Model file for the job. Use its own axes, mm. Give positions to 0.01 mm unless a question says otherwise; leave off trailing zeros. Order: outer loops, then holes, each group sorted by start corner. A loop starts at its lowest first (then second) coordinate and runs counter-clockwise, first axis right, second up. Notation, with made-up numbers: M 88,88 L 112,88 A25 ccw 112,111 Z; hole C -21.75,56.5 d1. An arc over 180 degrees is marked long. Return JSON: item names as keys, results as strings. Group by question number.
1. Slice it at B-B on z = 0. List the corners of the cut face in (x, y).
2. Slice it at D-D on z = -10. List the corners of the cut face in (x, y), then the cut area to 3 significant figures.
3. Pin check, flat tips, straight feed: pin 1 (2 mm diameter, centred on x = -8, y = -11.5, fed in from -Z); pin 2 (2.5 mm diameter, centred on x = -3.94, z = 6.82, fed in from +Y); pin 3 (4 mm diameter, centred on x = 4, y = -14.5, fed in from +Z); pin 4 (1 mm diameter, centred on y = -12, z = -9, fed in from -X). Stop position of each tip, or through.
4. Wall check: probe 1 along Z at (x, y) = (-3.25, -6.5); probe 2 along Z at (x, y) = (-2.75, -8.75); probe 3 along X at (y, z) = (-14.25, 5.75). Give the ranges that are in metal, low to high. Write a range as [from, to].
5. Slice it at C-C on x = 10.5. List the corners of the cut face in (y, z), then the cut area to 3 significant figures.
6. Two-plate mould, pull along X, no slides. Class faces 1 (the face through (-3.131, -10.14, 8.085)), 2 (the face through (-7.246, -9.86, 10.186)), 3 (the face through (6.377, -10.14, 0.066)), 4 (the face through (5.199, -9.86, 11.368)): released by +X, released by -X, zero draft, split by the parting line, or undercut.
7. Slice it at A-A on y = -16.5. List the corners of the cut face in (x, z).
from build123d import *

# Parameters (mm, degrees)
F1_DEPTH = 20
F3_D     = 3


with BuildPart() as f1:
    # F0 (on Front) → F1 (new body)
    with BuildSketch(Plane.XZ):
        Polygon((1.48048, -14.357629), (13.174312, -5.896681), (11.693831, 8.460948), (-1.48048, 14.357629), (-13.174312, 5.896681), (-11.693831, -8.460948), align=None)
    extrude(amount=F1_DEPTH)

    # F3 (through all)
    with Locations(Plane(origin=(0, 0, 0), x_dir=(-1, 0, 0), z_dir=(0, 1, 0))):
        with Locations((3.93769, -6.820278), (3.93769, 6.820278), (-7.875379, 0)):
            Hole(F3_D / 2)


solid = f1.part
Result:
{
 "1": {"outline": "M -12.57,-20 L 6.38,-20 L 6.38,0 L -12.57,0 Z; M 9.38,-20 L 12.57,-20 L 12.57,0 L 9.38,0 Z"},
 "2": {"outline": "M -8.26,-20 L 7.5,-20 L 7.5,0 L -8.26,0 Z", "area": "315 mm2"},
 "3": {"pin 1": "stops at z = -10.56", "pin 2": "passes through", "pin 3": "stops at z = 12.8", "pin 4": "stops at x = -11.61"},
 "4": {"probe 1": "z = [-12.24, -8.15], [-5.49, 5.49], [8.15, 13.08]", "probe 2": "z = [-12.46, -7.74], [-5.9, 5.9], [7.74, 13.44]", "probe 3": "x = [-13.16, -4.99], [-2.89, 11.97]"},
 "5": {"outline": "M -20,-7.83 L 0,-7.83 L 0,9 L -20,9 Z", "area": "337 mm2"},
 "6": {"face 1": "undercut", "face 2": "released by -X", "face 3": "undercut", "face 4": "released by +X"},
 "7": {"outline": "M -13.17,5.9 L -11.69,-8.46 L 1.48,-14.36 L 13.17,-5.9 L 11.69,8.46 L -1.48,14.36 Z; hole C -3.94,-6.82 d3; hole C -3.94,6.82 d3; hole C 7.88,0 d3"}
}
